Can you work these out from the model? Positions are in its coordinate system, mm. A direction names the side the tool comes from. Coordinates: 2 decimals unless noted, no trailing zeros. Loops run counter-clockwise (first coordinate to the right, second up) from the corner with the lowest first, then second, coordinate; pieces in that order, holes last.
```python
from build123d import *

# Parameters (mm, degrees)
BOSS_EXTRUDE1_DEPTH = 31.75
FILLET1_R           = 2.54
FILLET2_R           = 1.27
SKETCH2_R           = 6.35
CUT_EXTRUDE1_DEPTH  = 48.941448664
SKETCH3_R           = 2.4892
CUT_EXTRUDE2_DEPTH  = 47.33759959
SKETCH4_R           = 3.175
CUT_EXTRUDE3_DEPTH  = 47.337599597


with BuildPart() as part:
    # Sketch1 → Boss-Extrude1 (new body)
    with BuildSketch(Plane.XY):
        Polygon((0, 0), (0, 25.4), (3.175, 25.4), (3.175, 3.175), (25.4, 3.175), (25.4, 0), align=None)
    extrude(amount=BOSS_EXTRUDE1_DEPTH)

    # Fillet1
    fillet1_edges = [part.edges().sort_by_distance(p)[0] for p in [
        (3.175, 25.4, 15.875),
        (25.4, 3.175, 15.875),
    ]]
    fillet(fillet1_edges, radius=FILLET1_R)

    # Fillet2
    fillet2_edges = [part.edges().sort_by_distance(p)[0] for p in [
        (0, 0, 15.875),
        (3.175, 3.175, 15.875),
    ]]
    fillet(fillet2_edges, radius=FILLET2_R)

    # Sketch2 → Cut-Extrude1 (cut, through all)
    with BuildSketch(Plane.ZY):
        with Locations((15.875, 28.575)):
            Circle(SKETCH2_R)
    extrude(amount=-CUT_EXTRUDE1_DEPTH, mode=Mode.SUBTRACT)

    # Sketch3 → Cut-Extrude2 (cut, through all)
    with BuildSketch(Plane(origin=(0, 3.175, 0), x_dir=(1, 0, 0), z_dir=(0, 1, 0))):
        with Locations(Location((13.0175, -6.35, 0), (0, 0, 270))):
            Circle(SKETCH3_R)
        with Locations(Location((13.0175, -25.4, 0), (0, 0, 270))):
            Circle(SKETCH3_R)
    extrude(amount=-CUT_EXTRUDE2_DEPTH, mode=Mode.SUBTRACT)

    # Sketch4 → Cut-Extrude3 (cut, through all)
    with BuildSketch(Plane(origin=(3.175, 0, 0), x_dir=(0, 0, -1), z_dir=(1, 0, 0))):
        with Locations(Location((-15.875, 12.7, 0), (0, 0, 90))):
            Circle(SKETCH4_R)
    extrude(amount=-CUT_EXTRUDE3_DEPTH, mode=Mode.SUBTRACT)


solid = part.part
```
(1) I want a section at B-B on y = 12.7. Write out the boundary of the cut face in (x, z) (3 decimals), then the cut area to 3 significant figures.
Check values:
outline: (0, 0) - (3.175, 0) - (3.175, 12.7) - (0, 12.7) - close; (0, 19.05) - (3.175, 19.05) - (3.175, 31.75) - (0, 31.75) - close
area: 80.6 mm2
(2) I'm going to push flat-ended pins straight in: pin 1 (2 mm diameter, centred on x = 18, z = 24, fed in from +Y) (3 decimals); pin 2 (8 mm diameter, centred on x = 13.02, z = 25.4, fed in from -Y); pin 3 (5.5 mm diameter, centred on y = 14, z = 15, fed in from +X) (3 decimals); pin 4 (5 mm diameter, centred on x = 18.5, y = 6.5, fed in from -Z). Where does each tip first touch, or does it pass through?
Check values:
pin 1: stops at y = 3.175
pin 2: stops at y = 0
pin 3: stops at x = 3.175
pin 4: passes through
(3) If we mould it in two halves opening along Z, with no side actions, what happens to faces 3 (the cylindrical face through (15.116, 1.61, 7.688)), 4 (the cylindrical face through (2, 25, 5)), 5 (the flat face through (8, 2, 31.75))? For each: released by +Z, released by -Z, zero draft, split by the parting line, or undercut.
Check values:
face 3: undercut
face 4: zero draft
face 5: released by +Z
(4) Which directions (+Z, -Z, +X, -X, +Y, -Y) give clear straight access to the entire face, cutting with the end or side of a thin tool? Please do faces 1 (the flat face through (14, 0, 16)), 2 (the flat face through (14, 3.175, 16)).
Check values:
face 1: +Z, -Z, +X, -X, -Y
face 2: +Z, -Z, +X, +Y
(5) I want a section at A-A on z = 6.35. Write out the boundary of the cut face in (x, y) (3 decimals).
Check values:
outline: (0, 1.27) arc R1.27 ccw to (1.27, 0) - (10.528, 0) - (10.528, 3.175) - (4.445, 3.175) arc R1.27 cw to (3.175, 4.445) - (3.175, 22.86) arc R2.54 ccw to (0.635, 25.4) - (0, 25.4) - close; (15.507, 0) - (25.4, 0) - (25.4, 0.635) arc R2.54 ccw to (22.86, 3.175) - (15.507, 3.175) - close
(6) I want a section at C-C on x = 2.75. Write out the boundary of the cut face in (y, z) (3 decimals).
Check values:
outline: (0, 0) - (24.267, 0) - (24.267, 11.21) arc R6.35 cw to (24.267, 20.54) - (24.267, 31.75) - (0, 31.75) - close; hole circle Ø6.35 at (12.7, 15.875)
(7) If I drill on probe 1 along Z at (x, y) = (1.7, 12.7); probe 2 along X at (y, z) = (10.75, 24.5) (3 decimals), over which ranges is the centre line in solid material (lowest first)?
Check values:
probe 1: z = 0 to 12.7, 19.05 to 31.75
probe 2: x = 0 to 3.175
(8) I want a section at D-D on x = 9. Write out the boundary of the cut face in (y, z) (3 decimals), then the cut area to 3 significant figures.
Check values:
outline: (0, 0) - (3.175, 0) - (3.175, 31.75) - (0, 31.75) - close
area: 101 mm2
